from build123d import *

# Parameters (mm, degrees)
F1_DEPTH = 9
F2_R     = 8.74999
F3_R     = 4.5
F4_DEPTH = 6
F5_R     = 2


# Not quite as in the source:
# - a fillet or chamfer is up to 0.001 mm smaller than in the source, because OpenCascade refuses the exact size


with BuildPart() as f1:
    # F0 (on Top) → F1 (new body)
    with BuildSketch(Plane.XY):
        with BuildLine():
            Line((12.5, 8.75), (-12.5, 8.75))
            ThreePointArc((-12.5, 8.75), (-18.6871843354, 6.1871843354), (-21.25, 0))
            ThreePointArc((-21.25, 0), (-18.6871843354, -6.1871843354), (-12.5, -8.75))
            Line((-12.5, -8.75), (12.5, -8.75))
            ThreePointArc((12.5, -8.75), (18.6871843354, -6.1871843354), (21.25, 0))
            ThreePointArc((21.25, 0), (18.6871843354, 6.1871843354), (12.5, 8.75))
        make_face()
    extrude(amount=F1_DEPTH)

    # F2 (radius 8.75 in the source; OpenCascade refuses exactly that, so slightly less here)
    f2_edges = [f1.edges().sort_by_distance(p)[0] for p in [
        (21.25, 0, 0),
        (-21.25, 0, 0),
        (0, -8.75, 0),
        (0, 8.75, 0),
    ]]
    fillet(f2_edges, radius=F2_R)

    # F3 (on face) → F4 (join)
    with BuildSketch(Plane.XY.offset(9)):
        with Locations((12.5, 0)):
            Circle(F3_R)
        with Locations((-11.5, 0)):
            Circle(F3_R)
    extrude(amount=F4_DEPTH)

    # F5
    f5_edges = [f1.edges().sort_by_distance(p)[0] for p in [
        (-16, 0, 15),
        (8, 0, 15),
    ]]
    fillet(f5_edges, radius=F5_R)


solid = f1.part
Check sheet for the modelled part. Datum: model origin and axes. Units: mm. A direction names the side the tool comes from. Round coordinates to 2 decimals unless told otherwise and drop trailing zeros. Loops run counter-clockwise (first coordinate to the right, second up) from the corner with the lowest first, then second, coordinate; pieces in that order, holes last. Notation, with made-up numbers: (31, -24) - (63, -24) arc R36 ccw to (63, 14) - close; hole circle Ø2 at (68.25, 19). An arc over 180 degrees is marked (long way). Answer as CSV lines item,"result". Start each with the question number.
Item 1: Release check for a two-part mould opening along X. For faces 1 (the cylindrical face through (16.792, 1.352, 10.972)), 2 (the cylindrical face through (-0.175, 6.255, 2.631)) record: +X half, -X half, draft (parallel to the pull), parting line (faces both ways), or undercut.
Item 2: Depth check by flat-ended pin: P1, Ø3, axis at x = 4.5, y = 3, coming from the -Z side; P2, Ø1.5, axis at y = 6, z = 5, coming from the +X side; P3, Ø1.5, axis at x = 5.5, y = -5.5, coming from the -Z side. Enter the tip coordinate at first touch or a pass-through.
Item 3: Set-up check for faces 3 (the flat face through (-12, 0, 15)), 4 (the cylindrical face through (-7.208, 1.352, 10.972)): record each of +Z, -Z, +X, -X, +Y, -Y from which the full face is reachable in a straight line by a thin tool's end or side.
Item 4: Scan lines: line 1 (Y direction, x = -4, z = 8.5); line 2 (X direction, y = -2.5, z = 10.5); line 3 (Y direction, x = -6, z = 6.25). Record each from-to range of solid material in increasing order. Write a range as [from, to].
Item 5: Section check B-B (z = 11.25). Record the boundary of the cut face in (x, y), and give its area (3 significant figures).
Report:
1,face 1,"undercut"
1,face 2,"draft"
2,P1,"stops at z = 0.13"
2,P2,"stops at x = 18.55"
2,P3,"stops at z = 1.4"
3,face 3,"+Z, +X, -X, +Y, -Y"
3,face 4,"+Z"
4,line 1,"y = [-8.75, 8.75]"
4,line 2,"x = [-15.24, -7.76], [8.76, 16.24]"
4,line 3,"y = [-8.39, 8.39]"
5,outline,"circle Ø9 at (-11.5, 0); circle Ø9 at (12.5, 0)"
5,area,"127 mm2"
